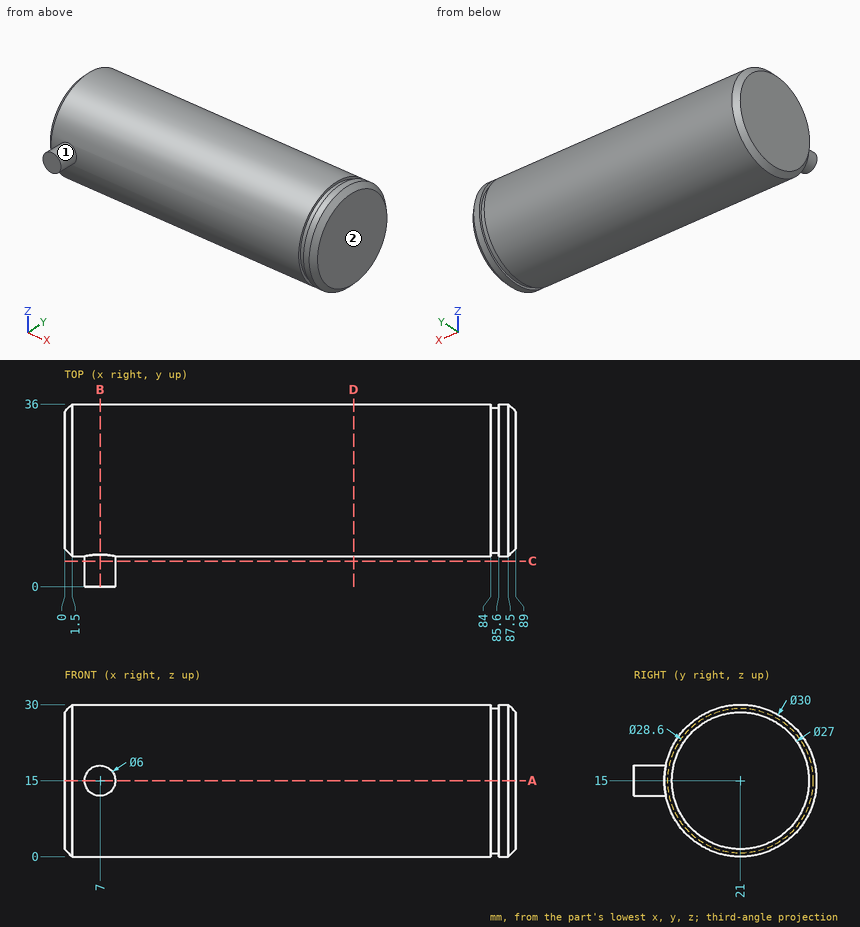
The figure shows three views and two pictorial views of one solid part (mm, origin at its lowest corner). Answer the questions. A direction names the side the tool comes from. Round coordinates to 2 decimals unless told otherwise and drop trailing zeros. Write each loop counter-clockwise with the first axis right and the second up, starting at its lowest first coordinate (ties: lowest second). Pieces come first, ordered by that corner, then holes. Notation, with made-up numbers: M -31.5,77.25 L 19.5,77.25 A21 ccw 19.5,108.25 Z; hole C 81.5,42 d6. An arc over 180 degrees is marked long. Write each question's results on one line, items separated by ' | '. Start each with the question number.
(1) For the marked faces 1 and 2, determine the directions among +Z, -Z, +X, -X, +Y, -Y from which every point of the face is accessible in a straight line to the end or side of a thin tool.
(2) Each of these flat-tipped pins is pushed along its axis until it touches: P1, Ø2, axis at x = 61.5, z = 23.5, coming from the +Y side; P2, Ø4, axis at y = 28.5, z = 13.5, coming from the -X side; P3, Ø2, axis at x = 37.5, y = 32.5, coming from the +Z side; P4, Ø12, axis at x = 9, y = 5, coming from the +Z side. Where does it stop, or does it pass through?
(3) Find the intervals of material crossed by line 1 (Z direction, x = 20, y = 14.5); line 2 (Y direction, x = 74.5, z = 3); line 3 (X direction, y = 29, z = 2.5), in increasing order.
(4) The part is cut by section A-A, the plane z = 15. Write down the section's boundary in (x, y), and give its area (3 significant figures).
(5) The part is cut by section D-D, the plane x = 57. Write down the section's boundary in (y, z).
(6) The part is cut by section C-C, the plane y = 5. Write down the section's boundary in (x, z).
(7) The part is cut by section B-B, the plane x = 7. Write down the section's boundary in (y, z), and give its area (3 significant figures).
Worked answers:
1) face 1: -Y | face 2: +Z, -Z, +X, +Y, -Y
2) P1: stops at y = 33.99 | P2: stops at x = 0 | P3: stops at z = 25.71 | P4: stops at z = 26.18
3) line 1: z = 1.48 to 28.52 | line 2: y = 12 to 30 | line 3: x = 1.34 to 84, 85.6 to 87.66
4) outline: M 0,7.5 L 1.5,6 L 4,6 L 4,0 L 10,0 L 10,6 L 84,6 L 84,6.7 L 85.6,6.7 L 85.6,6 L 87.5,6 L 89,7.5 L 89,34.5 L 87.5,36 L 85.6,36 L 85.6,35.3 L 84,35.3 L 84,36 L 1.5,36 L 0,34.5 Z | area: 2,700 mm²
5) outline: C 21,15 d30
6) outline: C 7,15 d6
7) outline: M 0,12 L 6.3,12 A15 ccw long 6.3,18 L 0,18 Z | area: 743 mm²
